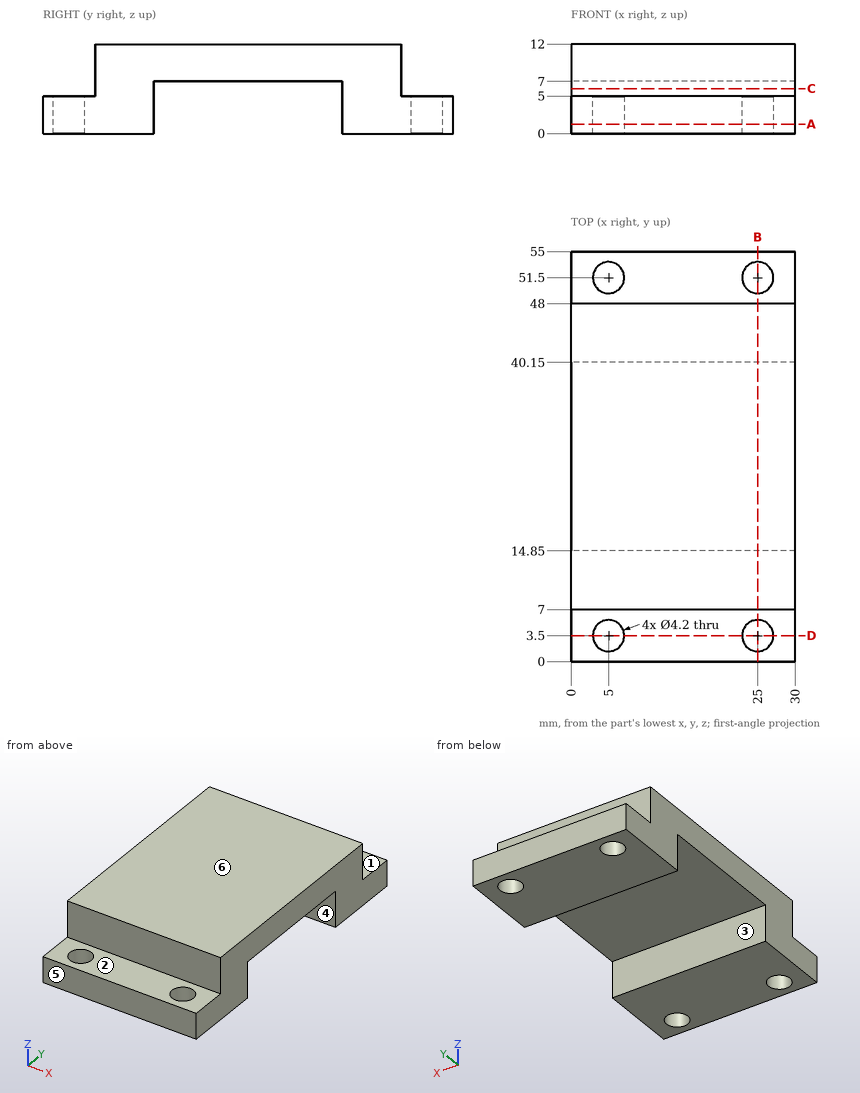
For this review, use the dimensioned drawing (mm, ordinates from the lowest corner) and the shaded views. A direction names the side the tool comes from. Round coordinates to 2 decimals unless told otherwise and drop trailing zeros. Write each loop counter-clockwise with the first axis right and the second up, starting at its lowest first coordinate (ties: lowest second). Pieces come first, ordered by that corner, then holes. Notation, with made-up numbers: M 69.25,80 L 86.25,80 A18 cw 86.25,95 Z; hole C -26.5,-8 d4. An arc over 180 degrees is marked long. Write item = value, one per line. Start each with the question number.
(1) We need section A-A (z = 1.25). Give the boundary of the cut face in (x, y).
(2) We need section D-D (y = 3.5). Give the boundary of the cut face in (x, z), then the cut area to 3 significant figures.
(3) We need section B-B (x = 25). Give the boundary of the cut face in (y, z).
(4) The part is to be moulded in two halves that separate along Y. For the marked faces 4, 5 and 6, say which applies: +Y half, -Y half, draft (parallel to the pull), parting line (faces both ways), or undercut.
(5) Clearance check with flat-ended pins moving along their axes: pin 1 Ø7.5 at (x, y) = (19.5, 51.5) entering from +Z; pin 2 Ø3.5 at (x, z) = (12, 8) entering from +Y; pin 3 Ø4 at (x, y) = (5, 51.5) entering from -Z (3 decimals); pin 4 Ø6.5 at (x, y) = (5, 3.5) entering from +Z. State where each tip first meets the part, or that it passes through.
(6) We need section C-C (z = 6). Give the boundary of the cut face in (x, y).
(7) For the marked faces 1, 2 and 3, list the 3-axis set-ups (+Z, -Z, +X, -X, +Y, -Y) from which the entire face can be reached by the end or side of a thin tool; tool diameter is ignored.
(8) For line 1 along Y through (x, z) = (25, 1.4); line 2 along Y through (x, z) = (23.5, 3.5); line 3 along Y through (x, z) = (21.25, 6.5), list the stretches that pass through material, from the lowest coordinate up.
Results found:
q1.outline = M 0,0 L 30,0 L 30,14.85 L 0,14.85 Z; M 0,40.15 L 30,40.15 L 30,55 L 0,55 Z; hole C 5,3.5 d4.2; hole C 5,51.5 d4.2; hole C 25,3.5 d4.2; hole C 25,51.5 d4.2
q2.outline = M 0,0 L 2.9,0 L 2.9,5 L 0,5 Z; M 7.1,0 L 22.9,0 L 22.9,5 L 7.1,5 Z; M 27.1,0 L 30,0 L 30,5 L 27.1,5 Z
q2.area = 108 mm²
q3.outline = M 0,0 L 1.4,0 L 1.4,5 L 0,5 Z; M 5.6,0 L 14.85,0 L 14.85,7 L 40.15,7 L 40.15,0 L 49.4,0 L 49.4,5 L 48,5 L 48,12 L 7,12 L 7,5 L 5.6,5 Z; M 53.6,0 L 55,0 L 55,5 L 53.6,5 Z
q4.face_4 = undercut
q4.face_5 = -Y half
q4.face_6 = draft
q5.pin_1 = 12
q5.pin_2 = 48
q5.pin_3 = through
q5.pin_4 = 5
q6.outline = M 0,7 L 30,7 L 30,14.85 L 0,14.85 Z; M 0,40.15 L 30,40.15 L 30,48 L 0,48 Z
q7.face_1 = +Z, +X, -X, +Y
q7.face_2 = +Z, +X, -X, -Y
q7.face_3 = -Z, +X, -X
q8.line_1 = 0 to 1.4, 5.6 to 14.85, 40.15 to 49.4, 53.6 to 55
q8.line_2 = 0 to 2.03, 4.97 to 14.85, 40.15 to 50.03, 52.97 to 55
q8.line_3 = 7 to 14.85, 40.15 to 48
